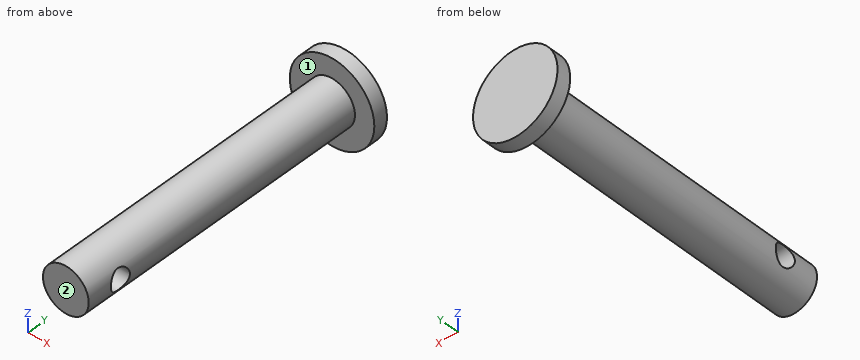
from build123d import *

# Parameters (mm, degrees)
F0_R     = 3.25
F1_DEPTH = 44
F0_R_2   = 6
F2_DEPTH = 2
F3_R     = 1.5
F4_DEPTH = 5


with BuildPart() as f1:
    # F0 (on Front) → F1 (new body)
    with BuildSketch(Plane.XZ):
        Circle(F0_R)
    extrude(amount=F1_DEPTH)

    # F0 (on Front) → F2 (join)
    with BuildSketch(Plane.XZ):
        Circle(F0_R_2)
        Circle(F0_R, mode=Mode.SUBTRACT)
    extrude(amount=F2_DEPTH)

    # F3 (on Right) → F4 (cut, symmetric)
    with BuildSketch(Plane.YZ):
        with Locations((-39, 0)):
            Circle(F3_R)
    extrude(amount=F4_DEPTH, both=True, mode=Mode.SUBTRACT)


solid = f1.part
Here's how the part is built. I have some questions about the finished solid (model axes, mm). Face numbers are marked on the shaded views. A direction names the side the tool comes from. Give positions to 0.01 mm unless a question says otherwise; leave off trailing zeros. Loops run counter-clockwise (first coordinate to the right, second up) from the corner with the lowest first, then second, coordinate; pieces in that order, holes last. Notation, with made-up numbers: (-11.75, 27.5) -> (39.25, 27.5) arc R12 cw to (39.25, 34.5) -> close; hole circle Ø1 at (77, 58). An arc over 180 degrees is marked (long way). One line per item, written item: value.
Q1. I'm going to push flat-ended pins straight in: pin 1 Ø1.5 at (y, z) = (-31.5, -0.5) entering from -X; pin 2 Ø1 at (x, y) = (1.5, -15.5) entering from +Z; pin 3 Ø1 at (y, z) = (-22, 1.5) entering from -X. Where does each tip first touch, or does it pass through?
Answers follow:
pin 1: x = -3.25
pin 2: z = 3.09
pin 3: x = -3.09
Q2. If I drill on line 1 along Y through (x, z) = (0.5, 0); line 2 along Z through (x, y) = (0.25, -39); line 3 along Y through (x, z) = (-1.25, -3.25), over which ranges is the centre line in solid material (lowest first)?
Answers follow:
line 1: -44 to -40.5, -37.5 to 0
line 2: -3.24 to -1.5, 1.5 to 3.24
line 3: -2 to 0
Q3. Suppose I cut it at B-B on x = 0. Please give me the cut outline in (y, z), then the cut area to 3 significant figures.
Answers follow:
outline: (-44, -3.25) -> (-2, -3.25) -> (-2, -6) -> (0, -6) -> (0, 6) -> (-2, 6) -> (-2, 3.25) -> (-44, 3.25) -> close; hole circle Ø3 at (-39, 0)
area: 290 mm^2
Q4. Suppose I cut it at D-D on x = -2.5. Please give me the cut outline in (y, z), then the cut area to 3 significant figures.
Answers follow:
outline: (-44, -2.08) -> (-2, -2.08) -> (-2, -5.45) -> (0, -5.45) -> (0, 5.45) -> (-2, 5.45) -> (-2, 2.08) -> (-44, 2.08) -> close; hole circle Ø3 at (-39, 0)
area: 189 mm^2
Q5. On a 3-axis mill with a long thin cutter (end or side, diameter ignored), from which of +Z, -Z, +X, -X, +Y, -Y can I reach the whole of each face in a straight line? I mean the marked faces 1 and 2. Say none if no direction works.
Answers follow:
face 1: -Y
face 2: +Z, -Z, +X, -X, -Y
Q6. Suppose I cut it at A-A on z = 0. Please give me the cut outline in (x, y).
Answers follow:
outline: (-6, -2) -> (-3.25, -2) -> (-3.25, -37.5) -> (3.25, -37.5) -> (3.25, -2) -> (6, -2) -> (6, 0) -> (-6, 0) -> close; (-3.25, -44) -> (3.25, -44) -> (3.25, -40.5) -> (-3.25, -40.5) -> close
Q7. Suppose I cut it at C-C on y = -39. Please give me the cut outline in (x, z), then the cut area to 3 significant figures.
Answers follow:
outline: (-2.88, -1.5) arc R3.25 ccw to (2.88, -1.5) -> close; (-2.88, 1.5) -> (2.88, 1.5) arc R3.25 ccw to start
area: 14.4 mm^2
